Part print with two shaded views. Sizes in mm from the minimum x, y, z corner. A direction names the side the tool comes from. Give positions to 0.01 mm unless a question says otherwise; leave off trailing zeros. Loops run counter-clockwise (first coordinate to the right, second up) from the corner with the lowest first, then second, coordinate; pieces in that order, holes last. Notation, with made-up numbers: M 17,-23.75 L 32,-23.75 A11 ccw 32,-4.75 Z; hole C -15,84 d9. An arc over 180 degrees is marked long. Answer as a JSON object with one key per item and string values. Group by question number.
1. Drill centre lines: line 1 along X through (y, z) = (7.75, 14.75) (1 decimal); line 2 along Z through (x, y) = (13.5, 5) (1 decimal); line 3 along X through (y, z) = (5, 7.75). Where is each one in solid material? Low to high. Write a range as [from, to].
2. Slice it at B-B (z = 11.25). List the corners of the cut face in (x, y).
3. Slice it at C-C (y = 1.25). List the corners of the cut face in (x, z) (1 decimal), then the cut area to 3 significant figures.
4. Mould opens along X. For the marked faces 1, 2 and 3 say: released by +X, released by -X, zero draft, split by the parting line, or undercut.
5. 3-axis set-ups, long thin cutter, end or side, ignore diameter. For the marked faces 4 and 5: which of +Z, -Z, +X, -X, +Y, -Y reach the whole face in a straight line?
6. Drop flat-ended pins along their axis: pin 1 Ø7.5 at (x, y) = (27, 8) entering from +Z (1 decimal); pin 2 Ø1 at (y, z) = (5.5, 12.5) entering from +X (1 decimal); pin 3 Ø6 at (x, z) = (8, 14.5) entering from -Y. Give the stop position or say it passes through.
7. Slice it at A-A (z = 5.5). List the corners of the cut face in (x, y).
8. Slice it at D-D (x = 38). List the corners of the cut face in (y, z) (1 decimal), then the cut area to 3 significant figures.
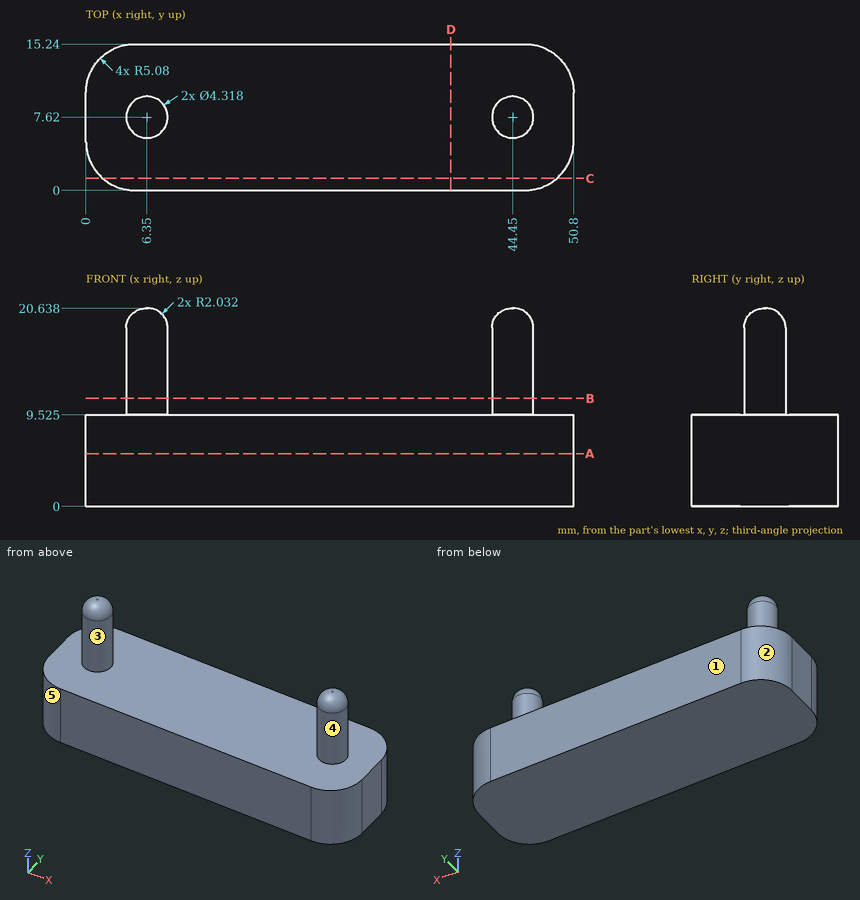
Established:
{
 "1": {"line 1": "x = [4.2, 8.5], [42.3, 46.6]", "line 2": "z = [0, 9.5]", "line 3": "x = [0, 50.8]"},
 "2": {"outline": "C 6.35,7.62 d4.32; C 44.45,7.62 d4.32"},
 "3": {"outline": "M 1.7,0 L 49.1,0 L 49.1,9.5 L 1.7,9.5 Z", "area": "451 mm^2"},
 "4": {"face 1": "zero draft", "face 2": "released by -X", "face 3": "undercut"},
 "5": {"face 4": "+Z", "face 5": "+Z, -Z, -X, -Y"},
 "6": {"pin 1": "stops at z = 9.5", "pin 2": "stops at x = 45.9", "pin 3": "stops at y = 5.46"},
 "7": {"outline": "M 0,5.08 A5.08 ccw 5.08,0 L 45.72,0 A5.08 ccw 50.8,5.08 L 50.8,10.16 A5.08 ccw 45.72,15.24 L 5.08,15.24 A5.08 ccw 0,10.16 Z"},
 "8": {"outline": "M 0,0 L 15.2,0 L 15.2,9.5 L 0,9.5 Z", "area": "145 mm^2"}
}
